```python
from build123d import *

# Parameters (mm, degrees)
BOSS_EXTRUDE1_DEPTH = 10
SKETCH2_R           = 2
SKETCH2_W           = 25
SKETCH2_H           = 55
CUT_EXTRUDE1_DEPTH  = 10


with BuildPart() as part:
    # Sketch1 → Boss-Extrude1 (new body)
    with BuildSketch(Plane(origin=(0, 0, 0), x_dir=(1, 0, 0), z_dir=(0, 1, 0))):
        Polygon((-75, 215), (-75, 135), (55, 135), (55, 0), (75, 0), (75, 215), (85, 215), (85, 315), (75, 315), (75, 560), (-75, 560), (-75, 315), (-85, 315), (-85, 215), align=None)
    extrude(amount=BOSS_EXTRUDE1_DEPTH)

    # Sketch2 → Cut-Extrude1 (cut)
    with BuildSketch(Plane(origin=(0, 10, 0), x_dir=(1, 0, 0), z_dir=(0, 1, 0))):
        with Locations((65, 10)):
            Circle(SKETCH2_R)
        with Locations((65, 460)):
            Circle(SKETCH2_R)
        with Locations((62.5, 532.5)):
            Rectangle(SKETCH2_W, SKETCH2_H)
    extrude(amount=-CUT_EXTRUDE1_DEPTH, mode=Mode.SUBTRACT)


solid = part.part
```
Here's how the part is built. I have some questions about the finished solid (model axes, mm). A direction names the side the tool comes from. Give positions to 0.01 mm unless a question says otherwise; leave off trailing zeros. Write each loop counter-clockwise with the first axis right and the second up, starting at its lowest first coordinate (ties: lowest second). Pieces come first, ordered by that corner, then holes. Notation, with made-up numbers: (-6.75, 83.5) -> (52.25, 83.5) arc R18 cw to (52.25, 118.5) -> close; hole circle Ø3 at (39.5, 6.25). An arc over 180 degrees is marked (long way). Write each question's results on one line, items separated by ' | '.
Item 1: Suppose I cut it at A-A on y = 3. Write out the boundary of the cut face in (x, z), plus the area to 4 significant figures.
Output:
outline: (-85, -315) -> (-75, -315) -> (-75, -560) -> (50, -560) -> (50, -505) -> (75, -505) -> (75, -315) -> (85, -315) -> (85, -215) -> (75, -215) -> (75, 0) -> (55, 0) -> (55, -135) -> (-75, -135) -> (-75, -215) -> (-85, -215) -> close; hole circle Ø4 at (65, -460); hole circle Ø4 at (65, -10) | area: 67,050 mm^2
Item 2: Suppose I cut it at B-B on x = -17. Write out the boundary of the cut face in (y, z).
Output:
outline: (0, -560) -> (10, -560) -> (10, -135) -> (0, -135) -> close
Item 3: For pin 1 Ø2 at (x, y) = (-48.5, 4) entering from +Z; pin 2 Ø5 at (y, z) = (3, -455) entering from -X; pin 3 Ø1.5 at (y, z) = (3.5, -62.5) entering from -X, each with a flat end and sliding along its axis, tell me the tip position at first contact or that it passes through.
Output:
pin 1: stops at z = -135 | pin 2: stops at x = -75 | pin 3: stops at x = 55
Item 4: On a 3-axis mill with a long thin cutter (end or side, diameter ignored), from which of +Z, -Z, +X, -X, +Y, -Y can I reach the whole of each face in a straight line? I mean faces 1 (the face through (62, 5, -505)), 2 (the face through (80, 5, -215)), 3 (the face through (-75, 5, -176)). Say none if no direction works.
Output:
face 1: -Z, +X, +Y, -Y | face 2: +Z, +X, +Y, -Y | face 3: +Z, -X, +Y, -Y
Item 5: Suppose I cut it at C-C on z = -423. Write out the boundary of the cut face in (x, y).
Output:
outline: (-75, 0) -> (75, 0) -> (75, 10) -> (-75, 10) -> close
Item 6: If I drill on L1, parallel to Z at x = 65, y = 4.5; L2, parallel to X at y = 5.25, z = -10; L3, parallel to X at y = 7, z = -460, over which ranges is the centre line in solid material (lowest first)?
Output:
L1: z = -505 to -462, -458 to -12, -8 to 0 | L2: x = 55 to 63, 67 to 75 | L3: x = -75 to 63, 67 to 75
